```python
from build123d import *

# Parameters (mm, degrees)
SKETCH1_R           = 4.01
BOSS_EXTRUDE1_DEPTH = 3
SKETCH2_R           = 1.49
BOSS_EXTRUDE3_DEPTH = 4
SKETCH4_W           = 10
SKETCH4_H           = 2.5
BOSS_EXTRUDE5_DEPTH = 15


with BuildPart() as part:
    # Sketch1 → Boss-Extrude1 (new body)
    with BuildSketch(Plane.XY):
        with BuildLine():
            Line((110, 10), (0, 10))
            ThreePointArc((0, 10), (-10, 0), (0, -10))
            Line((0, -10), (110, -10))
            ThreePointArc((110, -10), (120, 0), (110, 10))
        make_face()
        Circle(SKETCH1_R, mode=Mode.SUBTRACT)
        with Locations((110, 0)):
            Circle(SKETCH1_R, mode=Mode.SUBTRACT)
    extrude(amount=BOSS_EXTRUDE1_DEPTH)

    # Sketch2 → Boss-Extrude3 (add)
    with BuildSketch(Plane(origin=(0, 0, 0), x_dir=(-1, 0, 0), z_dir=(0, 0, -1))):
        with Locations(Location((-20, 0, 0), (0, 0, 180))):
            Circle(SKETCH2_R)
    extrude(amount=BOSS_EXTRUDE3_DEPTH)

    # Sketch4 → Boss-Extrude5 (add)
    with BuildSketch(Plane(origin=(0, 0, 0), x_dir=(-1, 0, 0), z_dir=(0, 0, -1))):
        with Locations((-0.046889456, 6.235161972)):
            Rectangle(SKETCH4_W, SKETCH4_H)
    extrude(amount=BOSS_EXTRUDE5_DEPTH)


solid = part.part
```
Verification items for the finished model (mm, model axes). A direction names the side the tool comes from. Give positions to 0.01 mm unless a question says otherwise; leave off trailing zeros. Loops run counter-clockwise (first coordinate to the right, second up) from the corner with the lowest first, then second, coordinate; pieces in that order, holes last.
1. Go/stop test with flat-tipped pins: pin 1 Ø12 at (x, y) = (17.5, -6.5) entering from -Z; pin 2 Ø0.8 at (y, z) = (7, -5) entering from +X; pin 3 Ø6.5 at (x, y) = (110, 0) entering from -Z; pin 4 Ø10 at (x, y) = (55.5, -3.5) entering from -Z. Record where each tip stops, or that it passes through.
2. Section check A-A, the plane y = 0. Enter the section's corners in (x, z), then the cut area to 3 significant figures.
3. Section check C-C, the plane x = 107.5. Enter the section's corners in (y, z), then the cut area to 3 significant figures.
4. Section check B-B, the plane x = 20. Enter the section's corners in (y, z).
5. Section check D-D, the plane y = -6.5. Enter the section's corners in (x, z), then the cut area to 3 significant figures.
6. Thickness scan on line 1 (Y direction, x = 110, z = 1.65); line 2 (X direction, y = 1.25, z = 2.25); line 3 (Z direction, x = 25, y = -6.75). Record the ranges inside material, lowest first.
7. Set-up check for faces 1 (the cylindrical face through (18.51, -0.07, -1.97)), 2 (the flat face through (5.047, 6, -7)), 3 (the flat face through (-4.953, 6, -7)): record each of +Z, -Z, +X, -X, +Y, -Y from which the full face is reachable in a straight line by a thin tool's end or side.
8. Mould release check, pull along Y, two halves, no side actions. Record for faces 4 (the cylindrical face through (105.994, 0.176, 1.479)), 5 (the flat face through (0, 7.485, -7)), 6 (the flat face through (0, 4.985, -7)): released by +Y, released by -Y, zero draft, split by the parting line, or undercut.
Geometry says:
1. pin 1: stops at z = -4
1. pin 2: stops at x = 5.05
1. pin 3: passes through
1. pin 4: stops at z = 0
2. outline: (-10, 0) - (-4.01, 0) - (-4.01, 3) - (-10, 3) - close; (4.01, 0) - (18.51, 0) - (18.51, -4) - (21.49, -4) - (21.49, 0) - (105.99, 0) - (105.99, 3) - (4.01, 3) - close; (114.01, 0) - (120, 0) - (120, 3) - (114.01, 3) - close
2. area: 354 mm2
3. outline: (-10, 0) - (-3.14, 0) - (-3.14, 3) - (-10, 3) - close; (3.14, 0) - (10, 0) - (10, 3) - (3.14, 3) - close
3. area: 41.2 mm2
4. outline: (-10, 0) - (-1.49, 0) - (-1.49, -4) - (1.49, -4) - (1.49, 0) - (10, 0) - (10, 3) - (-10, 3) - close
5. outline: (-7.6, 0) - (117.6, 0) - (117.6, 3) - (-7.6, 3) - close
5. area: 376 mm2
6. line 1: y = -10 to -4.01, 4.01 to 10
6. line 2: x = -9.92 to -3.81, 3.81 to 106.19, 113.81 to 119.92
6. line 3: z = 0 to 3
7. face 1: -Z
7. face 2: -Z, +X, +Y, -Y
7. face 3: -Z, -X, +Y, -Y
8. face 4: undercut
8. face 5: released by +Y
8. face 6: released by -Y
